Verification items for the finished model (mm, model axes). A direction names the side the tool comes from. Coordinates: 2 decimals unless noted, no trailing zeros. Order: outer loops, then holes, each group sorted by start corner. A loop starts at its lowest first (then second) coordinate and runs counter-clockwise, first axis right, second up. Notation, with made-up numbers: M 18.25,-33.75 L 69.25,-33.75 A11 cw 69.25,-19.75 Z; hole C -37,66 d1. An arc over 180 degrees is marked long. Answer as a JSON object with one key per item and string values. Group by question number.
(1) Access from +Z, -Z, +X, -X, +Y, -Y to the whole of each face (thin tool, end or side, straight path). Record for faces 1 (the face through (-0.54, 7.56, -8.48)), 2 (the face through (0, 1.5, 4.5)), 3 (the face through (7, 7, -2)).
(2) Cross-section at B-B (x = 0). Enter the section's corners in (y, z), plus the area to 3 significant figures.
(3) Cross-section at D-D (y = 1.75). Enter the section's corners in (x, z).
(4) Mould release check, pull along Z, two halves, no side actions. Record for faces 4 (the face through (2, 2, 0)), 5 (the face through (0, 6, -10)), 6 (the face through (0, 7, -7)), 7 (the face through (3, 3, 1)): released by +Z, released by -Z, zero draft, split by the parting line, or undercut.
(5) Gauge pin test, flat ends, axial feed: pin 1 Ø6 at (x, z) = (6.5, 1) entering from +Y; pin 2 Ø6.5 at (x, y) = (0, 10) entering from +Z; pin 3 Ø3 at (x, z) = (-7, 4) entering from +Y. Record the tip position at first contact, or that the pin passes through.
(6) Cross-section at A-A (y = 10). Enter the section's corners in (x, z).
(7) Material ranges on line 1 (Y direction, x = 0, z = -8.9); line 2 (X direction, y = 6.25, z = 6); line 3 (Z direction, x = 4.5, y = 8.75), recorded low to high.
(8) Cross-section at C-C (z = -0.5). Enter the section's corners in (x, y).
from build123d import *

# Parameters (mm, degrees)
SKETCH1_W           = 20
SKETCH1_H           = 20
BOSS_EXTRUDE1_DEPTH = 3
SKETCH2_W           = 20
SKETCH2_H           = 17
BOSS_EXTRUDE2_DEPTH = 3
BOSS_EXTRUDE3_DEPTH = 3
SKETCH4_R           = 2.5
CUT_EXTRUDE1_DEPTH  = 27.038433133
CUT_EXTRUDE2_DEPTH  = 4


with BuildPart() as part:
    # Sketch1 → Boss-Extrude1 (new body)
    with BuildSketch(Plane(origin=(0, 0, 0), x_dir=(1, 0, 0), z_dir=(0, 1, 0))):
        Rectangle(SKETCH1_W, SKETCH1_H)
    extrude(amount=BOSS_EXTRUDE1_DEPTH)

    # Sketch2 → Boss-Extrude2 (add)
    with BuildSketch(Plane(origin=(0, 0, -10), x_dir=(-1, 0, 0), z_dir=(0, 0, -1))):
        with Locations((0, 8.5)):
            Rectangle(SKETCH2_W, SKETCH2_H)
    extrude(amount=-BOSS_EXTRUDE2_DEPTH)

    # Sketch3 → Boss-Extrude3 (add)
    with BuildSketch(Plane(origin=(10, 0, 0), x_dir=(0, 0, -1), z_dir=(1, 0, 0))):
        Polygon((7, 17), (7, 3), (-10, 3), align=None)
    boss_extrude3 = extrude(amount=-BOSS_EXTRUDE3_DEPTH)

    # Mirror1: Boss-Extrude3 across plane
    add(boss_extrude3.mirror(Plane(origin=(0, 0, 0), x_dir=(0, 0, 1), z_dir=(1, 0, 0))))

    # Sketch4 → Cut-Extrude1 (cut, through all)
    with BuildSketch(Plane.XY.offset(-7)):
        with Locations((0, 10)):
            Circle(SKETCH4_R)
    extrude(amount=-CUT_EXTRUDE1_DEPTH, mode=Mode.SUBTRACT)

    # Sketch5 → Cut-Extrude2 (cut)
    with BuildSketch(Plane(origin=(0, 3, 0), x_dir=(1, 0, 0), z_dir=(0, 1, 0))):
        with BuildLine():
            Line((-2, -2.5), (-2, 2.5))
            ThreePointArc((-2, 2.5), (0, 4.5), (2, 2.5))
            Line((2, 2.5), (2, -2.5))
            ThreePointArc((2, -2.5), (0, -4.5), (-2, -2.5))
        make_face()
    extrude(amount=-CUT_EXTRUDE2_DEPTH, mode=Mode.SUBTRACT)


solid = part.part
Taken from the geometry:
{
 "1": {"face 1": "+Z, -Z", "face 2": "+Y, -Y", "face 3": "+Z, +Y"},
 "2": {"outline": "M 0,-10 L 7.5,-10 L 7.5,-7 L 3,-7 L 3,-4.5 L 0,-4.5 Z; M 0,4.5 L 3,4.5 L 3,10 L 0,10 Z; M 12.5,-10 L 17,-10 L 17,-7 L 12.5,-7 Z", "area": "60.0 mm²"},
 "3": {"outline": "M -10,-10 L 10,-10 L 10,10 L -10,10 Z; hole M -2,-2.5 A2 ccw 2,-2.5 L 2,2.5 A2 ccw -2,2.5 Z"},
 "4": {"face 4": "undercut", "face 5": "released by -Z", "face 6": "released by +Z", "face 7": "zero draft"},
 "5": {"pin 1": "stops at y = 12.85", "pin 2": "stops at z = -7", "pin 3": "stops at y = 9.18"},
 "6": {"outline": "M -10,-10 L -2.5,-10 L -2.5,-7 L -7,-7 L -7,1.5 L -10,1.5 Z; M 2.5,-10 L 10,-10 L 10,1.5 L 7,1.5 L 7,-7 L 2.5,-7 Z"},
 "7": {"line 1": "y = 0 to 7.5, 12.5 to 17", "line 2": "x = -10 to -7, 7 to 10", "line 3": "z = -10 to -7"},
 "8": {"outline": "M -10,0 L -2,0 L -2,3 L -7,3 L -7,11.65 L -10,11.65 Z; M 2,0 L 10,0 L 10,11.65 L 7,11.65 L 7,3 L 2,3 Z"}
}
